CAD build for the part. Positions are in the model's coordinates, mm. Face numbers are marked on the shaded views. A direction names the side the tool comes from. Round coordinates to 2 decimals unless told otherwise and drop trailing zeros. Loops run counter-clockwise (first coordinate to the right, second up) from the corner with the lowest first, then second, coordinate; pieces in that order, holes last. Notation, with made-up numbers: (28, 70) - (66, 70) arc R13 ccw to (66, 81) - close; hole circle Ø3 at (63, 78.25). An arc over 180 degrees is marked (long way). One line per question, with ' | ' between items.
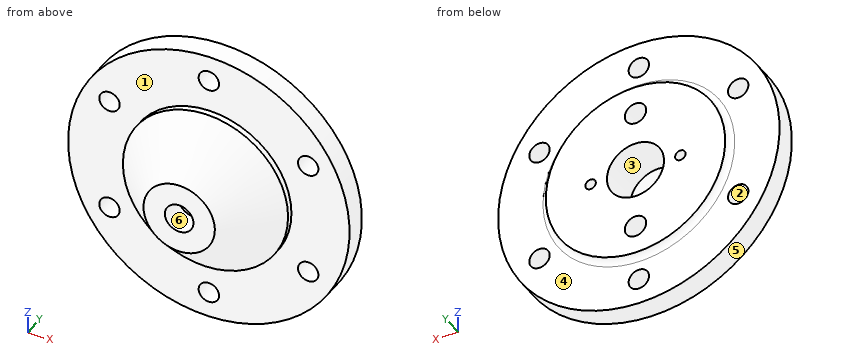
```python
from build123d import *

# Parameters (mm, degrees)
CUT_EXTRUDE1_REACH     = 211.077
SKETCH2_R              = 10
M24_TAPPED_HOLE1_D     = 21
M24_TAPPED_HOLE1_DEPTH = 27
M24_TAPPED_HOLE1_TIP   = 6.3090365
M12_TAPPED_HOLE1_D     = 10.2
M12_TAPPED_HOLE1_DEPTH = 50
M12_TAPPED_HOLE1_TIP   = 3.064389157


with BuildPart() as part:
    # Sketch1 → Revolve1 (revolve)
    with BuildSketch(Plane(origin=(0, 0, 0), x_dir=(0, 0, -1), z_dir=(1, 0, 0)), mode=Mode.PRIVATE) as revolve1_sk:
        with BuildLine():
            Line((14, 0), (35, 0))
            Line((35, 0), (81, 47))
            Line((81, 47), (81, 53))
            Line((81, 53), (138, 53))
            Line((138, 53), (138, 75))
            Line((138, 75), (94, 75))
            ThreePointArc((94, 75), (89.757359313, 76.757359313), (88, 81))
            Line((88, 81), (28, 81))
            Line((28, 81), (28, 39.304347826))
            Line((28, 39.304347826), (14, 25))
            Line((14, 25), (14, 0))
        make_face()
    revolve(revolve1_sk.sketch.rotate(Axis((0, 28, 0), (0, -1, 0)), 180), axis=Axis((0, 28, 0), (0, -1, 0)))

    # Sketch2 → Cut-Extrude1 (cut, up to next)
    with BuildSketch(Plane(origin=(0, 75, 0), x_dir=(1, 0, 0), z_dir=(0, 1, 0)), mode=Mode.PRIVATE) as cut_extrude1_sk1:
        with Locations(Location((0, 112.5, 0), (0, 0, 270))):
            Circle(SKETCH2_R)
    cut_extrude1_tool1 = extrude(cut_extrude1_sk1.sketch, amount=-CUT_EXTRUDE1_REACH, mode=Mode.PRIVATE) & part.part
    # Sketch2 → Cut-Extrude1 (cut, up to next)
    with BuildSketch(Plane(origin=(0, 75, 0), x_dir=(1, 0, 0), z_dir=(0, 1, 0)), mode=Mode.PRIVATE) as cut_extrude1_sk2:
        with Locations(Location((97.427857926, 56.25, 0), (0, 0, 270))):
            Circle(SKETCH2_R)
    cut_extrude1_tool2 = extrude(cut_extrude1_sk2.sketch, amount=-CUT_EXTRUDE1_REACH, mode=Mode.PRIVATE) & part.part
    # Sketch2 → Cut-Extrude1 (cut, up to next)
    with BuildSketch(Plane(origin=(0, 75, 0), x_dir=(1, 0, 0), z_dir=(0, 1, 0)), mode=Mode.PRIVATE) as cut_extrude1_sk3:
        with Locations(Location((97.427857926, -56.25, 0), (0, 0, 270))):
            Circle(SKETCH2_R)
    cut_extrude1_tool3 = extrude(cut_extrude1_sk3.sketch, amount=-CUT_EXTRUDE1_REACH, mode=Mode.PRIVATE) & part.part
    # Sketch2 → Cut-Extrude1 (cut, up to next)
    with BuildSketch(Plane(origin=(0, 75, 0), x_dir=(1, 0, 0), z_dir=(0, 1, 0)), mode=Mode.PRIVATE) as cut_extrude1_sk4:
        with Locations(Location((0, -112.5, 0), (0, 0, 270))):
            Circle(SKETCH2_R)
    cut_extrude1_tool4 = extrude(cut_extrude1_sk4.sketch, amount=-CUT_EXTRUDE1_REACH, mode=Mode.PRIVATE) & part.part
    # Sketch2 → Cut-Extrude1 (cut, up to next)
    with BuildSketch(Plane(origin=(0, 75, 0), x_dir=(1, 0, 0), z_dir=(0, 1, 0)), mode=Mode.PRIVATE) as cut_extrude1_sk5:
        with Locations(Location((-97.427857926, -56.25, 0), (0, 0, 270))):
            Circle(SKETCH2_R)
    cut_extrude1_tool5 = extrude(cut_extrude1_sk5.sketch, amount=-CUT_EXTRUDE1_REACH, mode=Mode.PRIVATE) & part.part
    # Sketch2 → Cut-Extrude1 (cut, up to next)
    with BuildSketch(Plane(origin=(0, 75, 0), x_dir=(1, 0, 0), z_dir=(0, 1, 0)), mode=Mode.PRIVATE) as cut_extrude1_sk6:
        with Locations(Location((-97.427857926, 56.25, 0), (0, 0, 270))):
            Circle(SKETCH2_R)
    cut_extrude1_tool6 = extrude(cut_extrude1_sk6.sketch, amount=-CUT_EXTRUDE1_REACH, mode=Mode.PRIVATE) & part.part
    add(cut_extrude1_tool1.solids().sort_by_distance((0, 75, -112.5))[0], mode=Mode.SUBTRACT)
    add(cut_extrude1_tool2.solids().sort_by_distance((97.427858, 75, -56.25))[0], mode=Mode.SUBTRACT)
    add(cut_extrude1_tool3.solids().sort_by_distance((97.427858, 75, 56.25))[0], mode=Mode.SUBTRACT)
    add(cut_extrude1_tool4.solids().sort_by_distance((0, 75, 112.5))[0], mode=Mode.SUBTRACT)
    add(cut_extrude1_tool5.solids().sort_by_distance((-97.427858, 75, 56.25))[0], mode=Mode.SUBTRACT)
    add(cut_extrude1_tool6.solids().sort_by_distance((-97.427858, 75, -56.25))[0], mode=Mode.SUBTRACT)

    # M24 Tapped Hole1
    with Locations(Plane(origin=(0, 81, -60), x_dir=(0, 0, 1), z_dir=(0, 1, 0))):
        with Locations((0, 0), (120, 0)):
            Hole(M24_TAPPED_HOLE1_D / 2, depth=M24_TAPPED_HOLE1_DEPTH)
            with Locations((0, 0, -(M24_TAPPED_HOLE1_DEPTH + M24_TAPPED_HOLE1_TIP / 2))):  # 118° drill point
                Cone(0, M24_TAPPED_HOLE1_D / 2, M24_TAPPED_HOLE1_TIP, mode=Mode.SUBTRACT)

    # M12 Tapped Hole1
    with Locations(Plane(origin=(44, 81, 0), x_dir=(0, 0, 1), z_dir=(0, 1, 0))):
        with Locations((0, 0), (0, -88)):
            Hole(M12_TAPPED_HOLE1_D / 2, depth=M12_TAPPED_HOLE1_DEPTH)
            with Locations((0, 0, -(M12_TAPPED_HOLE1_DEPTH + M12_TAPPED_HOLE1_TIP / 2))):  # 118° drill point
                Cone(0, M12_TAPPED_HOLE1_D / 2, M12_TAPPED_HOLE1_TIP, mode=Mode.SUBTRACT)


solid = part.part
```
(1) Cut at B-B, the plane y = 69.5. State how many separate pieces and enclosed holes the cut face has, then the cut area to 3 significant figures.
Results found:
separate pieces: 1 | enclosed holes: 11 | area: 54,600 mm²
(2) Drop flat-ended pins along their axis: P1, Ø4, axis at x = 0.5, z = 63, coming from the +Y side; P2, Ø4, axis at x = -12.5, z = -2, coming from the +Y side; P3, Ø10, axis at x = 88, z = -70, coming from the +Y side. Give the stop position or say it passes through.
Results found:
P1: stops at y = 50.72 | P2: stops at y = 25.67 | P3: stops at y = 75
(3) Cut at A-A, the plane z = 112.5. Write the cut outline in (x, y), then the cut area to 3 significant figures.
Results found:
outline: (-79.92, 53) - (-10, 53) - (-10, 75) - (-79.92, 75) - close; (10, 53) - (79.92, 53) - (79.92, 75) - (10, 75) - close | area: 3,080 mm²
(4) Two-plate mould, pull along Z, no slides. Class the marked faces 4, 5 and 6: released by +Z, released by -Z, zero draft, split by the parting line, or undercut.
Results found:
face 4: zero draft | face 5: split by the parting line | face 6: undercut
(5) Probe L1, parallel to X at y = 64.5, z = -60; L2, parallel to Y at x = 116.5, z = -27.5; L3, parallel to X at y = 56.5, z = -6. List the from-to ranges inside material, lowest first.
Results found:
L1: x = -124.27 to -106.7, -88.16 to -10.5, 10.5 to 88.16, 106.7 to 124.27 | L2: y = 53 to 75 | L3: x = -137.87 to -27.35, 27.35 to 137.87
(6) Tool access for the marked faces 1, 2 and 3: list every direction of +Z, -Z, +X, -X, +Y, -Y with a clear straight run to the whole face (end or side of a thin tool).
Results found:
face 1: -Y | face 2: +Y, -Y | face 3: +Y
